Geometry check sheet. Reference: the model listing, model coordinates, mm. Face numbers are marked on the shaded views. Give positions to 0.01 mm unless a question says otherwise; leave off trailing zeros. Loops run counter-clockwise (first coordinate to the right, second up) from the corner with the lowest first, then second, coordinate; pieces in that order, holes last. Notation, with made-up numbers: (-20.75, 9) -> (12.25, 9) arc R28 ccw to (12.25, 47) -> close; hole circle Ø11 at (68, 17). An arc over 180 degrees is marked (long way). Write each question's results on one line, items separated by ' | '. Start each with the question number.
1) Sectioned sample at D-D on y = 3.5. Record the cut outline in (x, z).
2) Sectioned sample at A-A on y = 10. Record the cut outline in (x, z), then the cut area to 3 significant figures.
3) Scan lines: line 1 (X direction, y = 10.75, z = 0.75); line 2 (Z direction, x = 3.25, y = 12.25); line 3 (X direction, y = 9.5, z = -0.25). Record each from-to range of solid material in increasing order. Write a range as from..to.
4) Depth check by flat-ended pin: pin 1 (1 mm diameter, centred on y = 2, z = 1, fed in from -X); pin 2 (1.6 mm diameter, centred on x = 0, z = 0, fed in from +Y); pin 3 (0.6 mm diameter, centred on x = 0, z = 0, fed in from -Y). Enter the tip coordinate at first touch or a pass-through.
5) Sectioned sample at C-C on z = 0.75. Record the cut outline in (x, y), then the cut area to 3 significant figures.
6) Sectioned sample at B-B on x = 0. Record the cut outline in (y, z).
7) Draft check along Z on the marked faces 1, 2, 3 and 4. Enter one of: pulls with the +Z half, pulls with the -Z half, needs draft (parallel to the pull), parting line crosses it, or undercut.
```python
from build123d import *

# Parameters (mm, degrees)
BOSS_EXTRUDE1_DEPTH = 12.73
SKETCH3_R           = 1.35255
CUT_EXTRUDE1_DEPTH  = 6
SKETCH4_R           = 0.353459893
CUT_EXTRUDE2_DEPTH  = 1


with BuildPart() as part:
    # Sketch1 → Boss-Extrude1 (new body)
    with BuildSketch(Plane(origin=(0, 0, 0), x_dir=(1, 0, 0), z_dir=(0, 1, 0))):
        Polygon((-4.618802154, 0), (-2.309401077, -4), (2.309401077, -4), (4.618802154, 0), (2.309401077, 4), (-2.309401077, 4), align=None)
    extrude(amount=BOSS_EXTRUDE1_DEPTH)

    # Sketch3 → Cut-Extrude1 (cut)
    with BuildSketch(Plane(origin=(0, 12.73, 0), x_dir=(1, 0, 0), z_dir=(0, 1, 0))):
        with Locations(Location((0, 0, 0), (0, 0, 270))):
            Circle(SKETCH3_R)
    extrude(amount=-CUT_EXTRUDE1_DEPTH, mode=Mode.SUBTRACT)

    # Sketch4 → Cut-Extrude2 (cut)
    with BuildSketch(Plane.XZ):
        with Locations(Location((0, 0, 0), (0, 0, 270))):
            Circle(SKETCH4_R)
    extrude(amount=-CUT_EXTRUDE2_DEPTH, mode=Mode.SUBTRACT)


solid = part.part
```
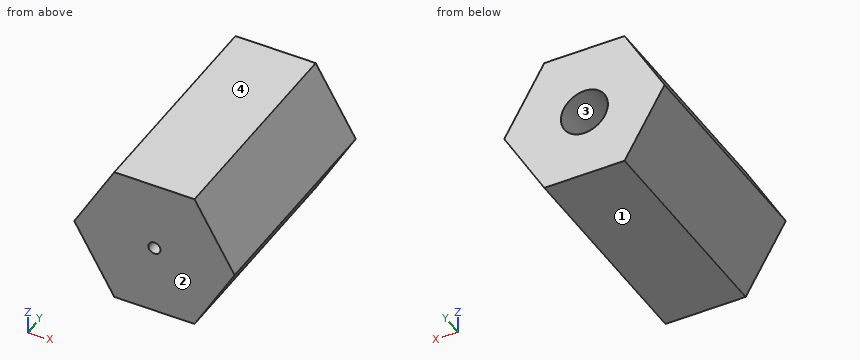
Result:
1) outline: (-4.62, 0) -> (-2.31, -4) -> (2.31, -4) -> (4.62, 0) -> (2.31, 4) -> (-2.31, 4) -> close
2) outline: (-4.62, 0) -> (-2.31, -4) -> (2.31, -4) -> (4.62, 0) -> (2.31, 4) -> (-2.31, 4) -> close; hole circle Ø2.71 at (0, 0) | area: 49.7 mm^2
3) line 1: -4.19..-1.13, 1.13..4.19 | line 2: -2.37..2.37 | line 3: -4.47..-1.33, 1.33..4.47
4) pin 1: x = -4.33 | pin 2: y = 6.73 | pin 3: y = 1
5) outline: (-4.19, 0) -> (4.19, 0) -> (4.19, 12.73) -> (1.13, 12.73) -> (1.13, 6.73) -> (-1.13, 6.73) -> (-1.13, 12.73) -> (-4.19, 12.73) -> close | area: 93.1 mm^2
6) outline: (0, -4) -> (12.73, -4) -> (12.73, -1.35) -> (6.73, -1.35) -> (6.73, 1.35) -> (12.73, 1.35) -> (12.73, 4) -> (0, 4) -> (0, 0.35) -> (1, 0.35) -> (1, -0.35) -> (0, -0.35) -> close
7) face 1: pulls with the -Z half | face 2: needs draft | face 3: undercut | face 4: pulls with the +Z half
